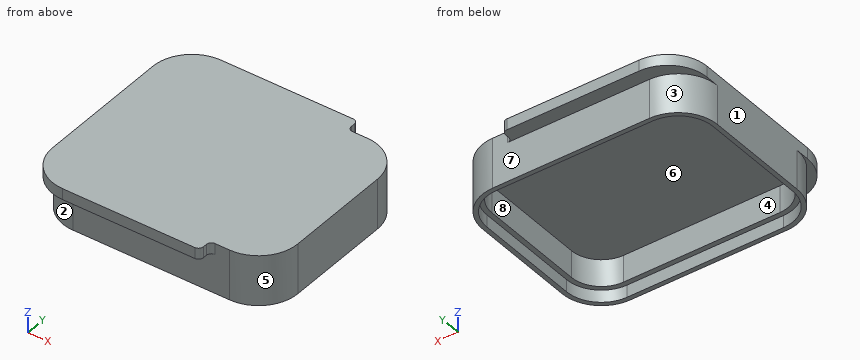
```python
from build123d import *

# Parameters (mm, degrees)
F1_DEPTH = 10.25
F2_W     = 36
F2_H     = 43.7
F3_DEPTH = 2.25
F4_R     = 8
F5_R     = 1
F6_R     = 1
F8_DEPTH = 8
F9_DEPTH = 2.5


with BuildPart() as f1:
    # F0 (on Top) → F1 (new body)
    with BuildSketch(Plane.XY):
        with BuildLine():
            Line((16, 19), (-16, 19))
            ThreePointArc((-16, 19), (-21.6568542495, 16.6568542495), (-24, 11))
            Line((-24, 11), (-24, -11))
            ThreePointArc((-24, -11), (-21.6568542495, -16.6568542495), (-16, -19))
            Line((-16, -19), (16, -19))
            ThreePointArc((16, -19), (21.6568542495, -16.6568542495), (24, -11))
            Line((24, -11), (24, 11))
            ThreePointArc((24, 11), (21.6568542495, 16.6568542495), (16, 19))
        make_face()
    extrude(amount=F1_DEPTH)

    # F2 (on face) → F3 (join)
    with BuildSketch(Plane.XY.offset(10.25)):
        with Locations((-6, 0)):
            Rectangle(F2_W, F2_H)
    extrude(amount=-F3_DEPTH)

    # F4
    f4_edges = [f1.edges().sort_by_distance(p)[0] for p in [
        (-24, -21.85, 9.125),
        (-24, 21.85, 9.125),
    ]]
    fillet(f4_edges, radius=F4_R)

    # F5
    f5_edges = [f1.edges().sort_by_distance(p)[0] for p in [
        (12, -21.85, 9.125),
        (12, 21.85, 9.125),
    ]]
    fillet(f5_edges, radius=F5_R)

    # F6
    f6_edges = [f1.edges().sort_by_distance(p)[0] for p in [
        (12, 19, 9.125),
        (12, -19, 9.125),
    ]]
    fillet(f6_edges, radius=F6_R)

    # F7 (on face) → F8 (cut)
    with BuildSketch(Plane(origin=(0, 0, 0), x_dir=(1, 0, 0), z_dir=(0, 0, -1))):
        with BuildLine():
            ThreePointArc((22.1, 11), (20.3133513652, 15.3133513652), (16, 17.1))
            Line((16, 17.1), (-16, 17.1))
            ThreePointArc((-16, 17.1), (-20.3133513652, 15.3133513652), (-22.1, 11))
            Line((-22.1, 11), (-22.1, -11))
            ThreePointArc((-22.1, -11), (-20.3133513652, -15.3133513652), (-16, -17.1))
            Line((-16, -17.1), (16, -17.1))
            ThreePointArc((16, -17.1), (20.3133513652, -15.3133513652), (22.1, -11))
            Line((22.1, -11), (22.1, 11))
        make_face()
    extrude(amount=-F8_DEPTH, mode=Mode.SUBTRACT)

    # F7 (on face) → F9 (cut)
    with BuildSketch(Plane(origin=(0, 0, 0), x_dir=(1, 0, 0), z_dir=(0, 0, -1))):
        with BuildLine():
            Line((23.1, -11), (23.1, 11))
            ThreePointArc((23.1, 11), (21.0204581464, 16.0204581464), (16, 18.1))
            Line((16, 18.1), (-16, 18.1))
            ThreePointArc((-16, 18.1), (-21.0204581464, 16.0204581464), (-23.1, 11))
            Line((-23.1, 11), (-23.1, -11))
            ThreePointArc((-23.1, -11), (-21.0204581464, -16.0204581464), (-16, -18.1))
            Line((-16, -18.1), (16, -18.1))
            ThreePointArc((16, -18.1), (21.0204581464, -16.0204581464), (23.1, -11))
        make_face()
        with BuildLine():
            Line((-16, 17.1), (16, 17.1))
            ThreePointArc((16, 17.1), (20.3133513652, 15.3133513652), (22.1, 11))
            Line((22.1, 11), (22.1, -11))
            ThreePointArc((22.1, -11), (20.3133513652, -15.3133513652), (16, -17.1))
            Line((16, -17.1), (-16, -17.1))
            ThreePointArc((-16, -17.1), (-20.3133513652, -15.3133513652), (-22.1, -11))
            Line((-22.1, -11), (-22.1, 11))
            ThreePointArc((-22.1, 11), (-20.3133513652, 15.3133513652), (-16, 17.1))
        make_face(mode=Mode.SUBTRACT)
    extrude(amount=-F9_DEPTH, mode=Mode.SUBTRACT)


solid = f1.part
```
The listing builds one solid part. Answer for the finished solid, in the listing's coordinates (mm). Face numbers are marked on the shaded views. A direction names the side the tool comes from. Give positions to 0.01 mm unless a question says otherwise; leave off trailing zeros. Order: outer loops, then holes, each group sorted by start corner. A loop starts at its lowest first (then second) coordinate and runs counter-clockwise, first axis right, second up.
Item 1: The part is cut by section D-D, the plane y = 2. Give the vertices of the cut face in (x, z).
From the geometry:
outline: (-24, 0) - (-23.1, 0) - (-23.1, 2.5) - (-22.1, 2.5) - (-22.1, 8) - (22.1, 8) - (22.1, 2.5) - (23.1, 2.5) - (23.1, 0) - (24, 0) - (24, 10.25) - (-24, 10.25) - close
Item 2: Which of the six approach directions +Z, -Z, +X, -X, +Y, -Y give full straight-line access (tool end or side, diameter ignored) to the marked faces 1, 2, 3 and 4?
From the geometry:
face 1: +Z, -Z, -X, +Y, -Y
face 2: -Z, -X, -Y
face 3: -Z, -X, +Y
face 4: -Z
Item 3: The part is cut by section A-A, the plane z = 6.25. Give the vertices of the cut face in (x, y), and give its area (3 significant figures).
From the geometry:
outline: (-24, -11) arc R8 ccw to (-16, -19) - (16, -19) arc R8 ccw to (24, -11) - (24, 11) arc R8 ccw to (16, 19) - (-16, 19) arc R8 ccw to (-24, 11) - close; hole (-22.1, -11) arc R6.1 ccw to (-16, -17.1) - (16, -17.1) arc R6.1 ccw to (22.1, -11) - (22.1, 11) arc R6.1 ccw to (16, 17.1) - (-16, 17.1) arc R6.1 ccw to (-22.1, 11) - close
area: 289 mm2
Item 4: The part is cut by section C-C, the plane z = 8.75. Give the vertices of the cut face in (x, y).
From the geometry:
outline: (-24, -13.85) arc R8 ccw to (-16, -21.85) - (11, -21.85) arc R1 ccw to (12, -20.85) - (12, -20) arc R1 cw to (13, -19) - (16, -19) arc R8 ccw to (24, -11) - (24, 11) arc R8 ccw to (16, 19) - (13, 19) arc R1 cw to (12, 20) - (12, 20.85) arc R1 ccw to (11, 21.85) - (-16, 21.85) arc R8 ccw to (-24, 13.85) - close
Item 5: For a pull along X with two mould halves and no side action, classify the marked faces 5, 6, 7 and 8 as pulls with the +X half, pulls with the -X half, needs draft (parallel to the pull), parting line crosses it, or undercut.
From the geometry:
face 5: pulls with the +X half
face 6: undercut
face 7: needs draft
face 8: undercut
Item 6: Find the intervals of material crossed by probe 1 along X at (y, z) = (2.5, 2); probe 2 along X at (y, z) = (-6, 6.25); probe 3 along Y at (x, z) = (9.5, 2.25), in increasing order.
From the geometry:
probe 1: x = -24 to -23.1, 23.1 to 24
probe 2: x = -24 to -22.1, 22.1 to 24
probe 3: y = -19 to -18.1, 18.1 to 19
Item 7: Given pin 1 Ø6 at (x, z) = (-5.5, 4) entering from -Y; pin 2 Ø3 at (x, z) = (6.5, 4) entering from +Y; pin 3 Ø1 at (y, z) = (13.5, 4.5) entering from -X, each flat-ended and moving along its own axis, determine where each tip first touches the part or whether it passes through.
From the geometry:
pin 1: stops at y = -19
pin 2: stops at y = 19
pin 3: stops at x = -23.75
Item 8: The part is cut by section B-B, the plane x = 14.5. Give the vertices of the cut face in (y, z).
From the geometry:
outline: (-19, 0) - (-18.1, 0) - (-18.1, 2.5) - (-17.1, 2.5) - (-17.1, 8) - (17.1, 8) - (17.1, 2.5) - (18.1, 2.5) - (18.1, 0) - (19, 0) - (19, 10.25) - (-19, 10.25) - close
